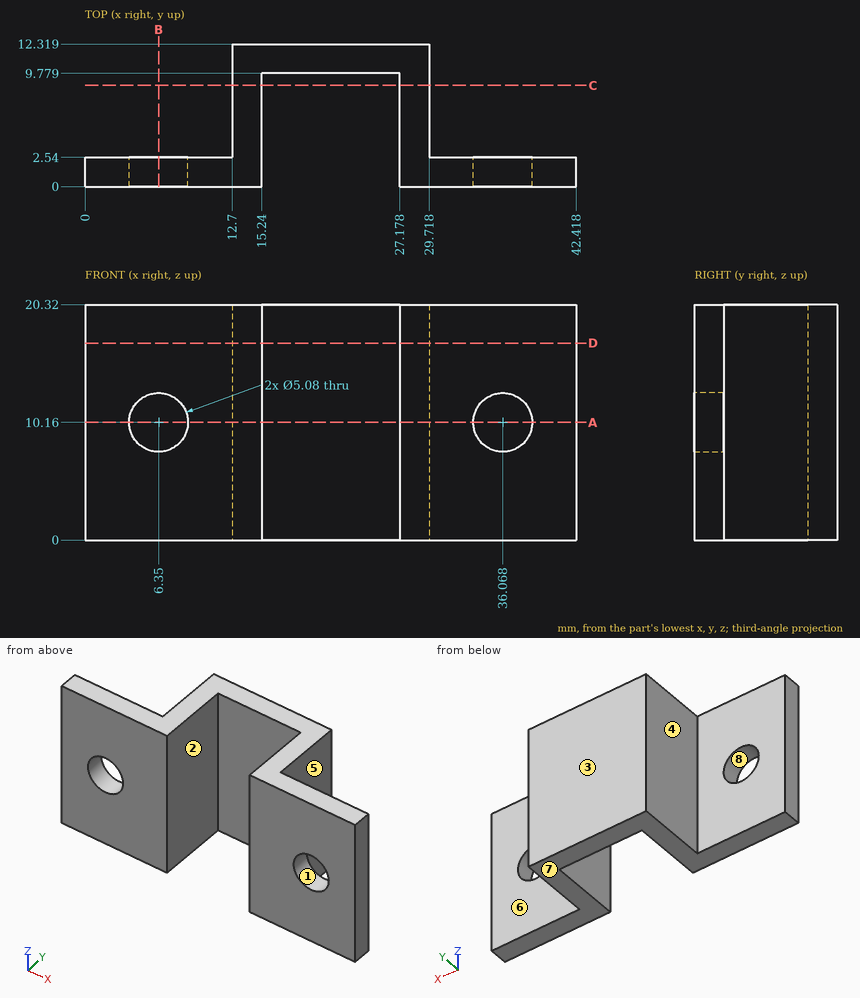
Print and shaded views of the part. All mm, measured from the part's lowest x, y and z. A direction names the side the tool comes from. Give positions to 0.01 mm unless a question says otherwise; leave off trailing zeros. Write each loop counter-clockwise with the first axis right and the second up, starting at its lowest first coordinate (ties: lowest second). Pieces come first, ordered by that corner, then holes. Notation, with made-up numbers: M -11,6 L 8,6 A23 ccw 8,17 Z; hole C 19,61 d9. An arc over 180 degrees is marked long. Use a Markdown table: item, result.
1) Cut at A-A (z = 10.16). List the corners of the cut face in (x, y), and give its area (3 significant figures).
Responses:
| item | result |
|---|---|
| outline | M 0,0 L 3.81,0 L 3.81,2.54 L 0,2.54 Z; M 8.89,0 L 15.24,0 L 15.24,9.78 L 27.18,9.78 L 27.18,0 L 33.53,0 L 33.53,2.54 L 29.72,2.54 L 29.72,12.32 L 12.7,12.32 L 12.7,2.54 L 8.89,2.54 Z; M 38.61,0 L 42.42,0 L 42.42,2.54 L 38.61,2.54 Z |
| area | 132 mm2 |
2) Pin check, flat tips, straight feed: pin 1 (2 mm diameter, centred on y = 5.5, z = 4, fed in from -X); pin 2 (6 mm diameter, centred on x = 36.068, z = 10.16, fed in from -Y); pin 3 (3 mm diameter, centred on x = 6.35, z = 10.16, fed in from -Y); pin 4 (1.5 mm diameter, centred on y = 7.5, z = 5.5, fed in from +X). Stop position of each tip, or through.
Responses:
| item | result |
|---|---|
| pin 1 | stops at x = 12.7 |
| pin 2 | stops at y = 0 |
| pin 3 | passes through |
| pin 4 | stops at x = 29.72 |
3) Cut at B-B (x = 6.35). List the corners of the cut face in (y, z).
Responses:
| item | result |
|---|---|
| outline | M 0,0 L 2.54,0 L 2.54,7.62 L 0,7.62 Z; M 0,12.7 L 2.54,12.7 L 2.54,20.32 L 0,20.32 Z |
4) Cut at D-D (z = 17). List the corners of the cut face in (x, y).
Responses:
| item | result |
|---|---|
| outline | M 0,0 L 15.24,0 L 15.24,9.78 L 27.18,9.78 L 27.18,0 L 42.42,0 L 42.42,2.54 L 29.72,2.54 L 29.72,12.32 L 12.7,12.32 L 12.7,2.54 L 0,2.54 Z |
5) Pull direction Z, two halves, no side cores. Call the marked faces 6, 7 and 8: +Z half, -Z half, draft (parallel to the pull), parting line (faces both ways), or undercut.
Responses:
| item | result |
|---|---|
| face 6 | draft |
| face 7 | -Z half |
| face 8 | undercut |
6) Tool access for the marked faces 1, 2, 3, 4 and 5: list every direction of +Z, -Z, +X, -X, +Y, -Y with a clear straight run to the whole face (end or side of a thin tool).
Responses:
| item | result |
|---|---|
| face 1 | +Y, -Y |
| face 2 | +Z, -Z, -Y |
| face 3 | +Z, -Z, +X, -X, +Y |
| face 4 | +Z, -Z, -X, +Y |
| face 5 | +Z, -Z, +X, +Y |
7) Drill centre lines: line 1 (X direction, y = 0.9, z = 10.16); line 2 (X direction, y = 2.25, z = 10.75); line 3 (X direction, y = 3.25, z = 11.25). Where is each one in solid material? Low to high. Write a range as from..to.
Responses:
| item | result |
|---|---|
| line 1 | x = 0..3.81, 8.89..15.24, 27.18..33.53, 38.61..42.42 |
| line 2 | x = 0..3.88, 8.82..15.24, 27.18..33.6, 38.54..42.42 |
| line 3 | x = 12.7..15.24, 27.18..29.72 |
8) Cut at C-C (y = 8.75). List the corners of the cut face in (x, z), and give its area (3 significant figures).
Responses:
| item | result |
|---|---|
| outline | M 12.7,0 L 15.24,0 L 15.24,20.32 L 12.7,20.32 Z; M 27.18,0 L 29.72,0 L 29.72,20.32 L 27.18,20.32 Z |
| area | 103 mm2 |
